from build123d import *

# Parameters (mm, degrees)
F0_R     = 1.5875
F1_DEPTH = 3.048


with BuildPart() as f1:
    # F0 (on Front) → F1 (new body)
    with BuildSketch(Plane.XZ):
        with BuildLine():
            Line((9.525, 0), (3.175, 0))
            ThreePointArc((3.175, 0), (-2.2450640303, -2.2450640303), (0, 3.175))
            Line((0, 3.175), (0, 9.525))
            ThreePointArc((0, 9.525), (-7.063929059, 6.3895642457), (-9.4772553384, -0.9525))
            ThreePointArc((-9.4772553384, -0.9525), (-6.3895642457, -7.063929059), (0, -9.525))
            Line((0, -9.525), (0.6773435479, -9.500885786))
            ThreePointArc((0.6773435479, -9.500885786), (6.9705567315, -6.4912990883), (9.525, 0))
        make_face()
        with BuildLine():
            ThreePointArc((0, 9.525), (6.7351920908, 6.7351920908), (9.525, 0))
            Line((9.525, 0), (36.5125, 0))
            ThreePointArc((36.5125, 0), (38.8373399243, 5.6126600757), (44.45, 7.9375))
            Line((44.45, 7.9375), (18.9664742022, 8.8511343208))
            ThreePointArc((18.9664742022, 8.8511343208), (13.260685791, 11.5695707689), (11.3409723165, 17.5912497948))
            Line((11.3409723165, 17.5912497948), (15.7954255641, 61.9125))
            ThreePointArc((15.7954255641, 61.9125), (10.6492737428, 51.7267849017), (0, 47.625))
            Line((0, 47.625), (0, 9.525))
        make_face()
        with BuildLine():
            Line((36.5125, 0), (9.525, 0))
            ThreePointArc((9.525, 0), (6.9705567315, -6.4912990883), (0.6773435479, -9.500885786))
            Line((0.6773435479, -9.500885786), (44.7324052746, -7.9324746146))
            ThreePointArc((44.7324052746, -7.9324746146), (38.9380895153, -5.7116327839), (36.5125, 0))
        make_face()
        with BuildLine():
            ThreePointArc((-9.4772553384, -0.9525), (-7.063929059, 6.3895642457), (0, 9.525))
            Line((0, 9.525), (0, 47.625))
            ThreePointArc((0, 47.625), (-10.6492737428, 51.7267849017), (-15.7954255641, 61.9125))
            Line((-15.7954255641, 61.9125), (-9.4772553384, -0.9525))
        make_face()
        with BuildLine():
            ThreePointArc((44.45, 7.9375), (38.8373399243, 5.6126600757), (36.5125, 0))
            ThreePointArc((36.5125, 0), (38.9380895153, -5.7116327839), (44.7324052746, -7.9324746146))
            ThreePointArc((44.7324052746, -7.9324746146), (50.1616327839, -5.5119104847), (52.3875, 0))
            ThreePointArc((52.3875, 0), (50.0626600757, 5.6126600757), (44.45, 7.9375))
        make_face()
        with BuildLine():
            ThreePointArc((47.625, 0), (44.45, -3.175), (41.275, 0))
            ThreePointArc((41.275, 0), (44.45, 3.175), (47.625, 0))
        make_face(mode=Mode.SUBTRACT)
        with BuildLine():
            ThreePointArc((0, -9.525), (0.3388863295, -9.5189695375), (0.6773435479, -9.500885786))
            Line((0.6773435479, -9.500885786), (0, -9.525))
        make_face()
        with BuildLine():
            Line((0, 60.325), (0, 47.625))
            ThreePointArc((0, 47.625), (10.6492737428, 51.7267849017), (15.7954255641, 61.9125))
            Line((15.7954255641, 61.9125), (14.9877324754, 68.7329246359))
            ThreePointArc((14.9877324754, 68.7329246359), (9.1908363712, 76.4438847259), (0, 79.375))
            Line((0, 79.375), (0, 66.675))
            ThreePointArc((0, 66.675), (2.2450640303, 65.7450640303), (3.175, 63.5))
            ThreePointArc((3.175, 63.5), (2.2450640303, 61.2549359697), (0, 60.325))
        make_face()
        with BuildLine():
            ThreePointArc((-15.7954255641, 61.9125), (-10.6492737428, 51.7267849017), (0, 47.625))
            Line((0, 47.625), (0, 60.325))
            ThreePointArc((0, 60.325), (-3.175, 63.5), (0, 66.675))
            Line((0, 66.675), (0, 79.375))
            ThreePointArc((0, 79.375), (-10.5003255158, 75.40625), (-15.7504882737, 65.484375))
            ThreePointArc((-15.7504882737, 65.484375), (-15.8737438155, 63.6997054867), (-15.7954255641, 61.9125))
        make_face()
        with BuildLine():
            Line((14.9877324754, 68.7329246359), (15.7954255641, 61.9125))
            ThreePointArc((15.7954255641, 61.9125), (15.8550939106, 62.7052534459), (15.875, 63.5))
            ThreePointArc((15.875, 63.5), (15.6516113875, 66.1538059417), (14.9877324754, 68.7329246359))
        make_face()
        with BuildLine():
            Line((-9.4502929642, 115.490625), (-15.7504882737, 65.484375))
            ThreePointArc((-15.7504882737, 65.484375), (-10.5003255158, 75.40625), (0, 79.375))
            Line((0, 79.375), (0, 104.775))
            ThreePointArc((0, 104.775), (-7.14375, 107.9998046905), (-9.4502929642, 115.490625))
        make_face()
        with Locations((-3.175, 100.0252)):
            Circle(F0_R, mode=Mode.SUBTRACT)
        with BuildLine():
            ThreePointArc((0, 79.375), (9.1908363712, 76.4438847259), (14.9877324754, 68.7329246359))
            Line((14.9877324754, 68.7329246359), (9.4589053806, 115.4201490977))
            ThreePointArc((9.4589053806, 115.4201490977), (9.5084619879, 114.8610486832), (9.525, 114.3))
            ThreePointArc((9.525, 114.3), (6.7351920908, 107.5648079092), (0, 104.775))
            Line((0, 104.775), (0, 79.375))
        make_face()
        with BuildLine():
            ThreePointArc((9.4589053806, 115.4201490977), (0.0355000934, 123.8249338446), (-9.4502929642, 115.490625))
            ThreePointArc((-9.4502929642, 115.490625), (-7.14375, 107.9998046905), (0, 104.775))
            ThreePointArc((0, 104.775), (6.7351920908, 107.5648079092), (9.525, 114.3))
            ThreePointArc((9.525, 114.3), (9.5084619879, 114.8610486832), (9.4589053806, 115.4201490977))
        make_face()
        with BuildLine():
            ThreePointArc((3.175, 114.3), (2.2450640303, 112.0549359697), (0, 111.125))
            ThreePointArc((0, 111.125), (-2.2450640303, 116.5450640303), (3.175, 114.3))
        make_face(mode=Mode.SUBTRACT)
    extrude(amount=F1_DEPTH)


solid = f1.part
The listing builds one solid part. Answer for the finished solid, in the listing's coordinates (mm). A direction names the side the tool comes from. Round coordinates to 2 decimals unless told otherwise and drop trailing zeros. Write each loop counter-clockwise with the first axis right and the second up, starting at its lowest first coordinate (ties: lowest second). Pieces come first, ordered by that corner, then holes. Notation, with made-up numbers: (48, 30) - (105, 30) arc R18 cw to (105, 55) - close; hole circle Ø8 at (69.25, 80). An arc over 180 degrees is marked (long way). Use a Markdown table: item, result. Add a question column.
1. Flat-ended cylindrical pins translate along their axes: P1, Ø1.5, axis at y = -1.5, z = 7.5, coming from the +X side; P2, Ø1.5, axis at x = 38.5, y = -0.5, coming from the -Z side; P3, Ø1.5, axis at y = -1.5, z = 66.5, coming from the +X side. Find the tip coordinate at first contact, or state that the pin passes through.
2. The part is cut by section A-A (x = 5). Write down the section's boundary in (y, z).
3. The part is cut by section B-B (y = -1.55). Give the number of separate pieces and of enclosed holes in the cut face, and give its area (3 significant figures).
4. The part is cut by section C-C (z = 89). Write down the section's boundary in (x, y), and give its area (3 significant figures).
5. For a pull along X with two mould halves and no side action, classify faces 3 (the face through (6.66, -1.5, 6.81)), 4 (the face through (13.537, -1.503, 39.442)), 5 (the face through (-15.873, -1.503, 63.725)) as +X half, -X half, draft (parallel to the pull), parting line (faces both ways), or undercut.
6. The part is cut by section D-D (x = 23). Write down the section's boundary in (y, z), and give its area (3 significant figures).
7. A tool of negligible diameter and unlimited length cuts with its end or side. For faces 1 (the face through (6, -2, 0)), 2 (the face through (52.387, -1.503, -0.031)), from which of +Z, -Z, +X, -X, +Y, -Y can it reach the whole face along a straight path? Write none if from no direction.
8. Consider line 1 (Z direction, x = 44.5, y = -2.65); line 2 (Z direction, x = 42, y = -1.05); line 3 (X direction, y = -1.8, z = 65). Determine where each line is inside the solid, lowest interval first.
Reported:
| question | item | result |
|---|---|---|
| 1 | P1 | x = 48.63 |
| 1 | P2 | z = -8.18 |
| 1 | P3 | x = 15.71 |
| 2 | outline | (-3.05, -9.35) - (0, -9.35) - (0, 0) - (-3.05, 0) - close; (-3.05, 8.11) - (0, 8.11) - (0, 122.41) - (-3.05, 122.41) - close |
| 3 | separate pieces | 1 |
| 3 | enclosed holes | 5 |
| 3 | area | 3,730 mm^2 |
| 4 | outline | (-12.79, -3.05) - (12.59, -3.05) - (12.59, 0) - (-12.79, 0) - close |
| 4 | area | 77.3 mm^2 |
| 5 | face 3 | undercut |
| 5 | face 4 | +X half |
| 5 | face 5 | -X half |
| 6 | outline | (-3.05, -8.71) - (0, -8.71) - (0, 8.71) - (-3.05, 8.71) - close |
| 6 | area | 53.1 mm^2 |
| 7 | face 1 | +Y, -Y |
| 7 | face 2 | +X, +Y, -Y |
| 8 | line 1 | -7.94 to -3.17, 3.17 to 7.94 |
| 8 | line 2 | -8.03 to -2.02, 2.02 to 8.03 |
| 8 | line 3 | -15.8 to -2.8, 2.8 to 15.8 |
